from build123d import *

# Parameters (mm, degrees)
TUBE_PLATE_MCP_BODY_DEPTH   = 2
TUBE_PLATE_MCP_CONTOURING_R = 1


with BuildPart() as part:
    # Sketch1 → Tube Plate MCP Body (new body)
    with BuildSketch(Plane.XY):
        with BuildLine():
            Line((-4.5, 0), (4.5, 0))
            Line((4.5, 0), (4.5, 2))
            Line((4.5, 2), (7.5, 2))
            Line((7.5, 2), (7.5, 5.75))
            Line((7.5, 5.75), (3.5, 5.75))
            Line((3.5, 5.75), (3.5, 4.75))
            ThreePointArc((3.5, 4.75), (2.5, 2.75), (1.5, 4.75))
            Line((1.5, 4.75), (1.5, 5.75))
            Line((1.5, 5.75), (-1.5, 5.75))
            Line((-1.5, 5.75), (-1.5, 4.75))
            ThreePointArc((-1.5, 4.75), (-2.5, 2.75), (-3.5, 4.75))
            Line((-3.5, 4.75), (-3.5, 5.75))
            Line((-3.5, 5.75), (-7.5, 5.75))
            Line((-7.5, 5.75), (-7.5, 2))
            Line((-7.5, 2), (-4.5, 2))
            Line((-4.5, 2), (-4.5, 0))
        make_face()
    extrude(amount=TUBE_PLATE_MCP_BODY_DEPTH)

    # Tube Plate MCP Contouring
    tube_plate_mcp_contouring_edges = [part.edges().sort_by_distance(p)[0] for p in [
        (-7.5, 5.75, 1),
        (7.5, 5.75, 1),
    ]]
    fillet(tube_plate_mcp_contouring_edges, radius=TUBE_PLATE_MCP_CONTOURING_R)


solid = part.part
Can you work these out from the model? Positions are in its coordinate system, mm. A direction names the side the tool comes from. Coordinates: 2 decimals unless noted, no trailing zeros. Loops run counter-clockwise (first coordinate to the right, second up) from the corner with the lowest first, then second, coordinate; pieces in that order, holes last. Notation, with made-up numbers: M 80,-19 L 100,-19 A25 ccw 100,1 Z; hole C 70,77 d1. An arc over 180 degrees is marked long. Answer as CSV lines item,"result". Start each with the question number.
1. Suppose I cut it at D-D, the plane x = 5.5. List the corners of the cut face in (y, z) for me, plus the area to 3 significant figures.
2. Suppose I cut it at C-C, the plane x = 2.5. List the corners of the cut face in (y, z) for me.
3. For pin 1 Ø0.6 at (y, z) = (1, 1) entering from -X; pin 2 Ø1.1 at (y, z) = (5.5, 0.5) entering from -X; pin 3 Ø0.8 at (y, z) = (5.5, 1) entering from -X; pin 4 Ø2 at (x, y) = (-2.5, 4) entering from +Z, each with a flat end and sliding along its axis, tell me the tip position at first contact or that it passes through.
4. Thinking about a two-plate mould opening in Y: for faces 1 (the face through (5, 5.75, 1)), 2 (the face through (-2.46, 2.75, 0.99)), 3 (the face through (4.5, 1, 1)), which applies, +Y half, -Y half, draft (parallel to the pull), parting line (faces both ways), or undercut?
5. If I drill on probe 1 along X at (y, z) = (3.25, 0.85); probe 2 along X at (y, z) = (5.3, 1.75); probe 3 along X at (y, z) = (1.75, 1.5), over which ranges is the centre line in solid material (lowest first)? Write a range as [from, to].
6. For faces 4 (the face through (6, 2, 1)), 5 (the face through (0, 5.75, 1)), 6 (the face through (-3.5, 5, 1)), 7 (the face through (-6, 2, 1)), which set-ups out of +Z, -Z, +X, -X, +Y, -Y let a thin tool reach every point of the face, with its end or its side?
7. Suppose I cut it at B-B, the plane z = 0.2. List the corners of the cut face in (x, y) for me, plus the area to 3 significant figures.
8. Suppose I cut it at A-A, the plane y = 4. List the corners of the cut face in (x, z) for me, plus the area to 3 significant figures.
Output:
1,outline,"M 2,0 L 5.75,0 L 5.75,2 L 2,2 Z"
1,area,"7.50 mm^2"
2,outline,"M 0,0 L 2.75,0 L 2.75,2 L 0,2 Z"
3,pin 1,"stops at x = -4.5"
3,pin 2,"stops at x = -7.48"
3,pin 3,"stops at x = -7.44"
3,pin 4,"passes through"
4,face 1,"+Y half"
4,face 2,"undercut"
4,face 3,"draft"
5,probe 1,"x = [-7.5, -3.5], [-1.5, 1.5], [3.5, 7.5]"
5,probe 2,"x = [-7.34, -3.5], [-1.5, 1.5], [3.5, 7.34]"
5,probe 3,"x = [-4.5, 4.5]"
6,face 4,"+Z, -Z, +X, -Y"
6,face 5,"+Z, -Z, +X, -X, +Y"
6,face 6,"+Z, -Z, +Y"
6,face 7,"+Z, -Z, -X, -Y"
7,outline,"M -7.5,2 L -4.5,2 L -4.5,0 L 4.5,0 L 4.5,2 L 7.5,2 L 7.5,4.75 A1 ccw 6.5,5.75 L 3.5,5.75 L 3.5,4.75 A1.25 cw long 1.5,4.75 L 1.5,5.75 L -1.5,5.75 L -1.5,4.75 A1.25 cw long -3.5,4.75 L -3.5,5.75 L -6.5,5.75 A1 ccw -7.5,4.75 Z"
7,area,"61.4 mm^2"
8,outline,"M -7.5,0 L -3.75,0 L -3.75,2 L -7.5,2 Z; M -1.25,0 L 1.25,0 L 1.25,2 L -1.25,2 Z; M 3.75,0 L 7.5,0 L 7.5,2 L 3.75,2 Z"
8,area,"20.0 mm^2"
